Study the drawing (mm; zero at the part's minimum x, y, z) and answer. Give positions to 0.01 mm unless a question says otherwise; leave off trailing zeros. Write each loop counter-clockwise with the first axis right and the second up, starting at its lowest first coordinate (ties: lowest second). Pieces come first, ordered by that corner, then holes. Notation, with made-up numbers: (10.25, 10.5) -> (66.25, 10.5) arc R21 ccw to (66.25, 20.5) -> close; hole circle Ø7 at (-9, 86). An arc over 180 degrees is marked (long way). One line per question, with ' | ' between items.
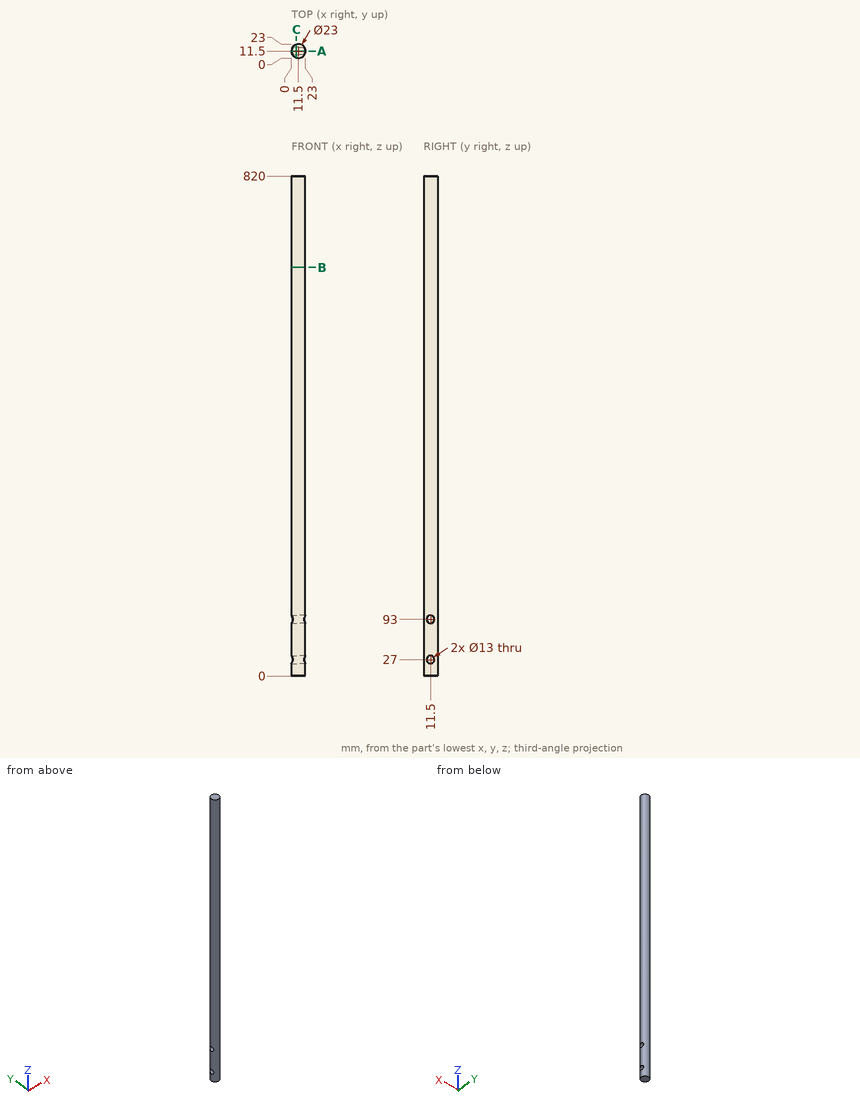
Item 1: Find section C-C (x = 8). Write down the section's boundary in (y, z).
Answers below:
outline: (0.55, 0) -> (22.45, 0) -> (22.45, 820) -> (0.55, 820) -> close; hole circle Ø13 at (11.5, 27); hole circle Ø13 at (11.5, 93)
Item 2: Find section B-B (z = 670). Write down the section's boundary in (x, y).
Answers below:
outline: circle Ø23 at (11.5, 11.5)
Item 3: Flat-ended cylindrical pins translate along their axes: pin 1 (1.5 mm diameter, centred on y = 20.5, z = 495, fed in from +X); pin 2 (8 mm diameter, centred on x = 6, z = 262.5, fed in from +Y); pin 3 (6 mm diameter, centred on y = 20, z = 396, fed in from +X). Find the tip coordinate at first contact, or state that the pin passes through.
Answers below:
pin 1: x = 19.51 | pin 2: y = 22.9 | pin 3: x = 21.6
Item 4: Find section A-A (y = 11.5). Write down the section's boundary in (x, z), then the cut area to 3 significant figures.
Answers below:
outline: (0, 0) -> (23, 0) -> (23, 20.5) -> (0, 20.5) -> close; (0, 33.5) -> (23, 33.5) -> (23, 86.5) -> (0, 86.5) -> close; (0, 99.5) -> (23, 99.5) -> (23, 820) -> (0, 820) -> close | area: 18,300 mm²
Item 5: Consider line 1 (Z direction, x = 8.5, y = 11.5); line 2 (Z direction, x = 9, y = 8.25); line 3 (Y direction, x = 10.25, z = 747.5). Determine where each line is inside the solid, lowest interval first. Write a range as [from, to].
Answers below:
line 1: [0, 20.5], [33.5, 86.5], [99.5, 820] | line 2: [0, 21.37], [32.63, 87.37], [98.63, 820] | line 3: [0.07, 22.93]
